Design review of the part built by this model. Coordinates are the model's own, in mm. Coordinates: 2 decimals unless noted, no trailing zeros. Write each loop counter-clockwise with the first axis right and the second up, starting at its lowest first coordinate (ties: lowest second). Pieces come first, ordered by that corner, then holes. Notation, with made-up numbers: (63.5, 76.25) - (76.5, 76.25) arc R6 ccw to (76.5, 85.25) - close; hole circle Ø10 at (10.25, -27). An arc over 180 degrees is marked (long way). Use a Markdown table: item, result.
from build123d import *

# Parameters (mm, degrees)
SKETCH1_R             = 1.5
SKETCH1_R_2           = 1.823358757
BOSS_EXTRUDE1_DEPTH   = 2
SKETCH1_W             = 69.213532985
SKETCH1_H             = 3
BOSS_EXTRUDE1_2_DEPTH = 2
SKETCH2_R             = 1.45
SKETCH2_R_2           = 1.449999997
BOSS_EXTRUDE2_DEPTH   = 5
SKETCH3_R             = 2.5
BOSS_EXTRUDE3_DEPTH   = 1


with BuildPart() as part:
    # Sketch1 → Boss-Extrude1 (new body)
    with BuildSketch(Plane(origin=(0, 0, 0), x_dir=(1, 0, 0), z_dir=(0, 1, 0))):
        with BuildLine():
            Line((40.328427125, 26.5), (40.328427125, 23.5))
            ThreePointArc((40.328427125, 23.5), (38.533566599, 21.320123126), (35.739793711, 21.730270106))
            Line((35.739793711, 21.730270106), (-0.120981949, 3.988623195))
            Line((-0.120981949, 3.988623195), (-35.707345562, 21.594508352))
            ThreePointArc((-35.707345562, 21.594508352), (-38.6168059, 21.215624921), (-40.458039892, 23.5))
            Line((-40.458039892, 23.5), (-40.458039892, 26.5))
            Line((-40.458039892, 26.5), (-49, 26.5))
            ThreePointArc((-49, 26.5), (-54.974873735, 28.974873735), (-52.5, 23))
            Line((-52.5, 23), (-52.5, 0))
            Line((-52.5, 0), (-52.5, -26.5))
            Line((-52.5, -26.5), (-40.328427125, -26.5))
            Line((-40.328427125, -26.5), (-40.328427125, -23.5))
            ThreePointArc((-40.328427125, -23.5), (-38.560823049, -21.693818527), (-36.040421728, -21.879001857))
            Line((-36.040421728, -21.879001857), (0.120981949, -3.988623195))
            Line((0.120981949, -3.988623195), (39.558871233, -23.5))
            Line((39.558871233, -23.5), (-34.671572875, -23.5))
            Line((-34.671572875, -23.5), (-34.671572875, -26.5))
            Line((-34.671572875, -26.5), (-7, -26.5))
            Line((-7, -26.5), (-7, -31.5))
            Line((-7, -31.5), (5, -31.5))
            Line((5, -31.5), (5, -26.5))
            Line((5, -26.5), (42.041960109, -26.5))
            Line((42.041960109, -26.5), (42.041960109, -24.5))
            Line((42.041960109, -24.5), (42.041960108, -24.395234694))
            Line((42.041960109, -24.395234694), (42.041960109, -23.5))
            ThreePointArc((42.041960109, -23.5), (45, -21.377501001), (47.958039892, -23.5))
            Line((47.958039892, -23.5), (47.958039892, -26.5))
            Line((47.958039892, -26.5), (50.5, -26.5))
            Line((50.5, -26.5), (50.5, -25.302775638))
            Line((50.5, -25.302775638), (50.5, 22.341687605))
            Line((50.5, 22.341687605), (50.5, 23))
            ThreePointArc((50.5, 23), (52.974873734, 28.974873734), (47, 26.5))
            Line((47, 26.5), (40.328427125, 26.5))
        make_face()
        Polygon((8.062110713, -0.059854228), (47.5, 19.451522577), (47.5, -19.571231035), (42.041960107, -16.870937614), align=None, mode=Mode.SUBTRACT)
        with Locations(Location((-3.5, -29, 0), (0, 0, 270))):
            Circle(SKETCH1_R, mode=Mode.SUBTRACT)
        with Locations(Location((1.5, -29, 0), (0, 0, 270))):
            Circle(SKETCH1_R, mode=Mode.SUBTRACT)
        Polygon((-8.062110713, 0.059854228), (-47.5, -19.451522577), (-47.5, 19.571231035), align=None, mode=Mode.SUBTRACT)
        with Locations(Location((-52.5, 26.5, 0), (0, 0, 270))):
            Circle(SKETCH1_R_2, mode=Mode.SUBTRACT)
        with Locations(Location((50.5, 26.5, 0), (0, 0, 270))):
            Circle(SKETCH1_R, mode=Mode.SUBTRACT)
    extrude(amount=BOSS_EXTRUDE1_DEPTH)



with BuildPart() as body_2:
    # Sketch1 → Boss-Extrude1 2 (new body)
    with BuildSketch(Plane(origin=(0, 0, 0), x_dir=(1, 0, 0), z_dir=(0, 1, 0))):
        with Locations((0.064806384, 25)):
            Rectangle(SKETCH1_W, SKETCH1_H)
    extrude(amount=BOSS_EXTRUDE1_2_DEPTH)


with BuildPart() as part_1:
    add(part.part)

    add(body_2.part)  # Boss-Extrude2 merges body 2
    # Sketch2 → Boss-Extrude2 (add)
    # profile 1 of 4: a face of its own
    with BuildSketch(Plane(origin=(0, 0, 0), x_dir=(1, 0, 0), z_dir=(0, 1, 0))):
        with BuildLine():
            ThreePointArc((-34.671572875, -23.5), (-37.5, -21.5), (-40.328427125, -23.5))
            Line((-40.328427125, -23.5), (-40.328427125, -26.5))
            Line((-40.328427125, -26.5), (-34.671572875, -26.5))
            Line((-34.671572875, -26.5), (-34.671572875, -23.5))
        make_face()
        with Locations(Location((-37.5, -24.5, 0), (0, 0, 270))):
            Circle(SKETCH2_R, mode=Mode.SUBTRACT)
    # profile 2 of 4: a face of its own
    with BuildSketch(Plane(origin=(0, 0, 0), x_dir=(1, 0, 0), z_dir=(0, 1, 0))):
        with BuildLine():
            Line((-40.458039892, 26.5), (-40.458039892, 23.5))
            ThreePointArc((-40.458039892, 23.5), (-37.5, 21), (-34.541960108, 23.5))
            Line((-34.541960108, 23.5), (-34.541960108, 26.5))
            Line((-34.541960108, 26.5), (-40.458039892, 26.5))
        make_face()
        with Locations(Location((-37.5, 24, 0), (0, 0, 270))):
            Circle(SKETCH2_R, mode=Mode.SUBTRACT)
    # profile 3 of 4: a face of its own
    with BuildSketch(Plane(origin=(0, 0, 0), x_dir=(1, 0, 0), z_dir=(0, 1, 0))):
        with BuildLine():
            ThreePointArc((47.958039892, -23.5), (45, -21.377501001), (42.041960109, -23.5))
            Line((42.041960109, -23.5), (42.041960109, -26.5))
            Line((42.041960109, -26.5), (47.397915762, -26.5))
            Line((47.397915762, -26.5), (47.958039892, -26.5))
            Line((47.958039892, -26.5), (47.958039892, -23.5))
        make_face()
        with Locations(Location((45, -24.5, 0), (0, 0, 270))):
            Circle(SKETCH2_R, mode=Mode.SUBTRACT)
    # profile 4 of 4: a face of its own
    with BuildSketch(Plane(origin=(0, 0, 0), x_dir=(1, 0, 0), z_dir=(0, 1, 0))):
        with BuildLine():
            Line((40.328427125, 26.5), (34.671572877, 26.5))
            Line((34.671572877, 26.5), (34.671572877, 23.5))
            ThreePointArc((34.671572877, 23.5), (37.500000001, 21.127718682), (40.328427125, 23.5))
            Line((40.328427125, 23.5), (40.328427125, 24))
            Line((40.328427125, 24), (40.328427125, 26.5))
        make_face()
        with Locations(Location((37.500000001, 24.000000006, 0), (0, 0, 270))):
            Circle(SKETCH2_R_2, mode=Mode.SUBTRACT)
    extrude(amount=BOSS_EXTRUDE2_DEPTH)

    # Sketch3 → Boss-Extrude3 (add)
    with BuildSketch(Plane(origin=(0, 0, 0), x_dir=(1, 0, 0), z_dir=(0, 1, 0))):
        with Locations((-52.5, -26.5)):
            Circle(SKETCH3_R)
    extrude(amount=BOSS_EXTRUDE3_DEPTH)


solid = part_1.part
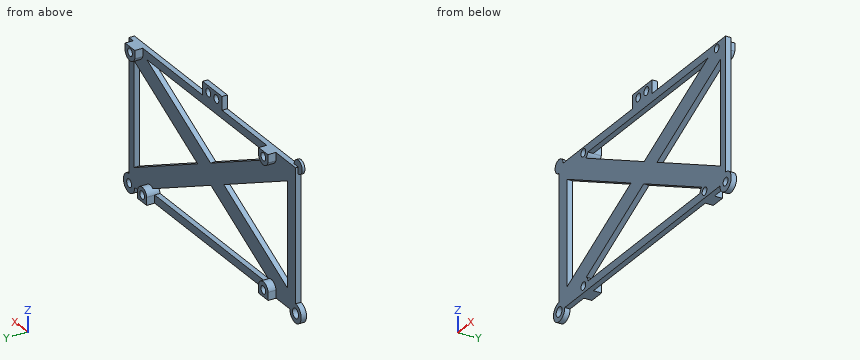
(1) For L1, parallel to X at y = 2.15, z = 24.5; L2, parallel to X at y = 1, z = 29; L3, parallel to X at y = 2.65, z = -24, list the stretches that pass through material, from the lowest coordinate up. Write a range as from..to.
Determined:
| item | result |
|---|---|
| L1 | -40.33..-38.95, -36.05..-34.67, 42.04..43.55, 46.45..47.96 |
| L2 | -7..-5, -2..0, 3..5 |
| L3 | -40.46..-38.95, -36.05..-34.54, 34.67..36.05, 38.95..40.33 |
(2) Take a section at A-A on y = 3.85. State how many separate pieces and enclosed holes the cut face has, and give its area (3 significant figures).
Determined:
| item | result |
|---|---|
| separate pieces | 4 |
| enclosed holes | 4 |
| area | 81.7 mm2 |
(3) For pin 1 (2.5 mm diameter, centred on y = 4, z = 24.5, fed in from +X); pin 2 (1.5 mm diameter, centred on x = 37, y = 0.5, fed in from -Z); pin 3 (1 mm diameter, centred on y = 1.5, z = -9, fed in from -X), all flat-tipped, find the tip position at first contact; note any pin that passes through.
Determined:
| item | result |
|---|---|
| pin 1 | x = 47.96 |
| pin 2 | z = -26.5 |
| pin 3 | x = -52.5 |
(4) Take a section at B-B on x = -43. Write out the cut boundary in (y, z).
Determined:
| item | result |
|---|---|
| outline | (0, -26.5) - (2, -26.5) - (2, -17.34) - (0, -17.34) - close; (0, 17.23) - (2, 17.23) - (2, 26.5) - (0, 26.5) - close |
(5) Take a section at C-C on x = -3.5. Write out the cut boundary in (y, z), and give its area (3 significant figures).
Determined:
| item | result |
|---|---|
| outline | (0, -26.5) - (2, -26.5) - (2, -23.5) - (0, -23.5) - close; (0, -5.66) - (2, -5.66) - (2, 5.78) - (0, 5.78) - close; (0, 23.5) - (2, 23.5) - (2, 27.5) - (0, 27.5) - close; (0, 30.5) - (2, 30.5) - (2, 31.5) - (0, 31.5) - close |
| area | 38.9 mm2 |
